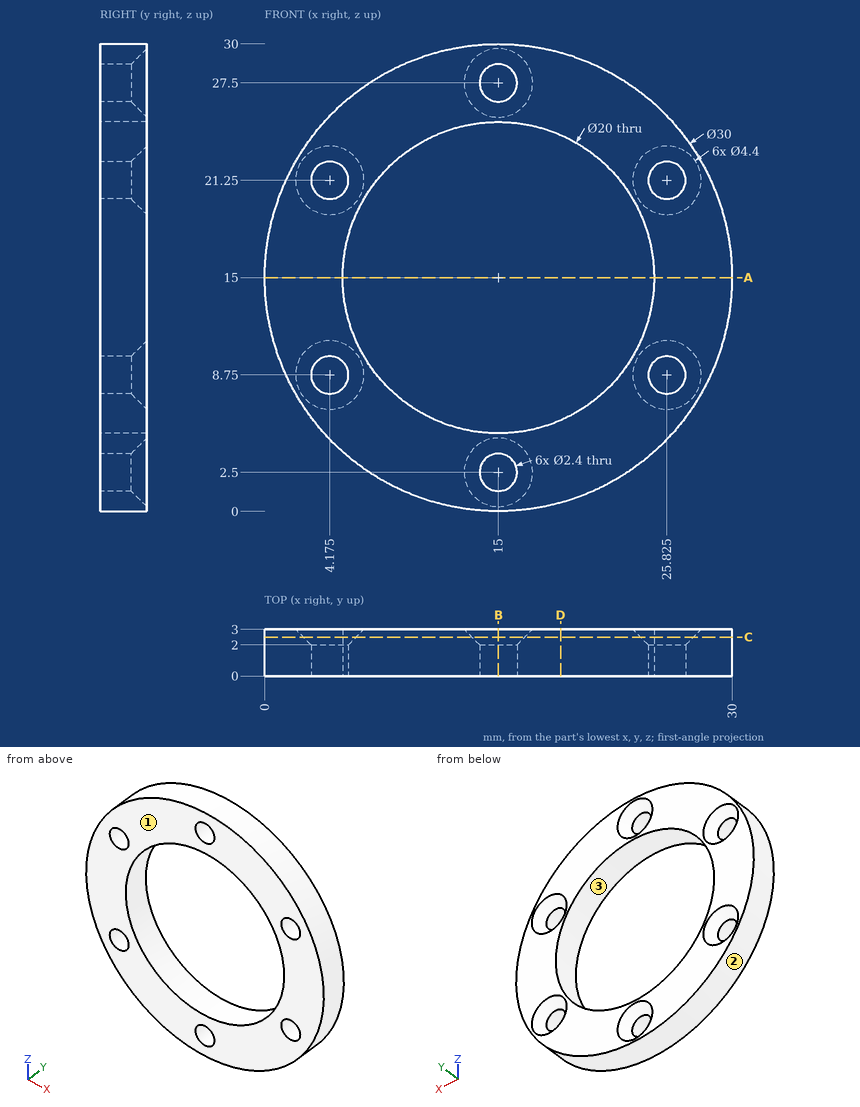
Here's the drawing with two shaded views (mm, measured from the low corner). I have some questions. Give positions to 0.01 mm unless a question says otherwise; leave off trailing zeros. Loops run counter-clockwise (first coordinate to the right, second up) from the corner with the lowest first, then second, coordinate; pieces in that order, holes last. Notation, with made-up numbers: M -3,59 L 12,59 A36 ccw 12,98 Z; hole C 5.5,-7 d3. An arc over 180 degrees is marked long. Use one line per item in the form item = value. Start each with the question number.
(1) Thinking about a two-plate mould opening in Z: for the marked faces 1, 2 and 3, which applies, released by +Z, released by -Z, zero draft, split by the parting line, or undercut?
(2) Please list where these lines run through material, in increasing order: line 1 (Z direction, x = 26, y = 0.1); line 2 (Z direction, x = 3.75, y = 1.45); line 3 (X direction, y = 1, z = 8.5).
(3) I'm going to push flat-ended pins straight in: P1, Ø1, axis at y = 2, z = 21, coming from the -X side (1 decimal); P2, Ø3, axis at x = 15, z = 27.5, coming from the +Y side; P3, Ø4, axis at x = 25.83, z = 21.25, coming from the +Y side (1 decimal); P4, Ø12, axis at x = 26.5, z = 5.5, coming from the -Y side. Where does each tip first touch, or does it pass through?
(4) I want a section at B-B, the plane x = 15. Write out the boundary of the cut face in (y, z), and give its area (3 significant figures).
(5) I want a section at A-A, the plane z = 15. Write out the boundary of the cut face in (x, y), and give its area (3 significant figures).
(6) I want a section at D-D, the plane x = 19. Write out the boundary of the cut face in (y, z) (1 decimal).
(7) I want a section at C-C, the plane y = 2.5. State how many separate pieces and enclosed holes the cut face has, and give its area (3 significant figures).
Worked out:
q1.face_1 = zero draft
q1.face_2 = split by the parting line
q1.face_3 = undercut
q2.line_1 = 4.8 to 7.56, 9.94 to 20.06, 22.44 to 25.2
q2.line_2 = 5.08 to 7.63, 9.87 to 20.13, 22.37 to 24.92
q2.line_3 = 1.48 to 3, 5.35 to 7.4, 22.6 to 24.65, 27 to 28.52
q3.P1 = 1
q3.P2 = 2.3
q3.P3 = 2.8
q3.P4 = 0
q4.outline = M 0,0 L 3,0 L 3,0.3 L 2,1.3 L 0,1.3 Z; M 0,3.7 L 2,3.7 L 3,4.7 L 3,5 L 0,5 Z; M 0,25 L 3,25 L 3,25.3 L 2,26.3 L 0,26.3 Z; M 0,28.7 L 2,28.7 L 3,29.7 L 3,30 L 0,30 Z
q4.area = 13.6 mm²
q5.outline = M 0,0 L 5,0 L 5,3 L 0,3 Z; M 25,0 L 30,0 L 30,3 L 25,3 Z
q5.area = 30.0 mm²
q6.outline = M 0,0.5 L 3,0.5 L 3,5.8 L 0,5.8 Z; M 0,24.2 L 3,24.2 L 3,29.5 L 0,29.5 Z
q7.separate_pieces = 1
q7.enclosed_holes = 7
q7.area = 338 mm²
